Work out the finished part from the listing and answer in its coordinate system (mm). A direction names the side the tool comes from. Round coordinates to 2 decimals unless told otherwise and drop trailing zeros. Loops run counter-clockwise (first coordinate to the right, second up) from the corner with the lowest first, then second, coordinate; pieces in that order, holes last. Notation, with made-up numbers: (-10.75, 74) - (11.25, 74) arc R30 ccw to (11.25, 105) - close; hole circle Ø3 at (54.25, 85). An arc over 180 degrees is marked (long way). Return JSON: item names as keys, results as strings.
from build123d import *

# Parameters (mm, degrees)
SKETCH_1_W          = 100
SKETCH_1_H          = 11.5
EXTRUDE_1_DEPTH     = 3
SKETCH_2_W          = 2.5
SKETCH_2_H          = 11.5
EXTRUDE_2_DEPTH     = 26
SKETCH_3_W          = 2.5
SKETCH_3_H          = 11.5
EXTRUDE_3_DEPTH     = 20
SKETCH_6_W          = 2.5
SKETCH_6_H          = 16.5
EXTRUDE_4_DEPTH     = 8
CUT_EXTRUDE_1_DEPTH = 101


with BuildPart() as part:
    # 草图1 → 凸台-拉伸1 (new body)
    with BuildSketch(Plane(origin=(0, 0, 0), x_dir=(1, 0, 0), z_dir=(0, 1, 0))):
        with Locations((50, 5.75)):
            Rectangle(SKETCH_1_W, SKETCH_1_H)
    extrude(amount=EXTRUDE_1_DEPTH)

    # 草图2 → 凸台-拉伸2 (add)
    with BuildSketch(Plane(origin=(0, 3, 0), x_dir=(1, 0, 0), z_dir=(0, 1, 0))):
        with Locations((1.25, 5.75)):
            Rectangle(SKETCH_2_W, SKETCH_2_H)
        with Locations((98.75, 5.75)):
            Rectangle(SKETCH_2_W, SKETCH_2_H)
    extrude(amount=EXTRUDE_2_DEPTH)

    # 草图3 → 凸台-拉伸3 (add)
    with BuildSketch(Plane(origin=(0, 3, 0), x_dir=(1, 0, 0), z_dir=(0, 1, 0))):
        with Locations((22.25, 5.75)):
            Rectangle(SKETCH_3_W, SKETCH_3_H)
        with Locations((77.75, 5.75)):
            Rectangle(SKETCH_3_W, SKETCH_3_H)
    extrude(amount=EXTRUDE_3_DEPTH)

    # 草图6 → 凸台-拉伸4 (add)
    with BuildSketch(Plane(origin=(0, 29, 0), x_dir=(1, 0, 0), z_dir=(0, 1, 0))):
        with Locations((1.25, 5.75)):
            Rectangle(SKETCH_6_W, SKETCH_6_H)
        with Locations((98.75, 5.75)):
            Rectangle(SKETCH_6_W, SKETCH_6_H)
    extrude(amount=EXTRUDE_4_DEPTH)

    # 草图5 → 切除-拉伸1 (cut, through all)
    with BuildSketch(Plane(origin=(100, 0, 0), x_dir=(0, 0, -1), z_dir=(1, 0, 0))):
        Polygon((8.25, 31.165063509), (7, 33.330127019), (4.5, 33.330127019), (3.25, 31.165063509), (4.5, 29), (7, 29), align=None)
    extrude(amount=-CUT_EXTRUDE_1_DEPTH, mode=Mode.SUBTRACT)


solid = part.part
1) Section B-B (z = -9.5) is taken. Give the vertices of the cut face in (x, y), and give its area (3 significant figures).
Verdict:
{"outline": "(0, 0) - (100, 0) - (100, 37) - (97.5, 37) - (97.5, 3) - (79, 3) - (79, 23) - (76.5, 23) - (76.5, 3) - (23.5, 3) - (23.5, 23) - (21, 23) - (21, 3) - (2.5, 3) - (2.5, 37) - (0, 37) - close", "area": "570 mm2"}
2) Section A-A (y = 34.5) is taken. Give the vertices of the cut face in (x, z).
Verdict:
{"outline": "(0, -14) - (2.5, -14) - (2.5, 2.5) - (0, 2.5) - close; (97.5, -14) - (100, -14) - (100, 2.5) - (97.5, 2.5) - close"}
3) Section C-C (y = 13) is taken. Give the vertices of the cut face in (x, z).
Verdict:
{"outline": "(0, -11.5) - (2.5, -11.5) - (2.5, 0) - (0, 0) - close; (21, -11.5) - (23.5, -11.5) - (23.5, 0) - (21, 0) - close; (76.5, -11.5) - (79, -11.5) - (79, 0) - (76.5, 0) - close; (97.5, -11.5) - (100, -11.5) - (100, 0) - (97.5, 0) - close"}
4) Find the intervals of material crossed by L1, parallel to X at y = 16.5, z = -0.5; L2, parallel to X at y = 31.5, z = -9.25; L3, parallel to Y at x = 30.5, z = -7.25, in increasing order.
Verdict:
{"L1": "x = 0 to 2.5, 21 to 23.5, 76.5 to 79, 97.5 to 100", "L2": "x = 0 to 2.5, 97.5 to 100", "L3": "y = 0 to 3"}
5) A tool of negligible diameter and unlimited length cuts with its end or side. For faces 3 (the flat face through (88, 3, -6)), 4 (the flat face through (1.267, 32.232, -7.634)), 5 (the flat face through (99, 29, -13)), from which of +Z, -Z, +X, -X, +Y, -Y can it reach the whole face along a straight path? Write none if from no direction.
Verdict:
{"face 3": "+Z, -Z, +Y", "face 4": "+X, -X", "face 5": "-Z, +X, -X, -Y"}
6) Flat-ended cylindrical pins translate along their axes: pin 1 (10 mm diameter, centred on x = 30, y = 20, fed in from +Z); pin 2 (6 mm diameter, centred on x = 15.5, z = -6.5, fed in from +Y); pin 3 (0.8 mm diameter, centred on x = 22, z = -6, fed in from +Y); pin 4 (0.8 mm diameter, centred on x = 99, z = -12.5, fed in from -Y). Find the tip coordinate at first contact, or state that the pin passes through.
Verdict:
{"pin 1": "passes through", "pin 2": "stops at y = 3", "pin 3": "stops at y = 23", "pin 4": "stops at y = 29"}
7) Section D-D (x = 66.5) is taken. Give the vertices of the cut face in (y, z), and give its area (3 significant figures).
Verdict:
{"outline": "(0, -11.5) - (3, -11.5) - (3, 0) - (0, 0) - close", "area": "34.5 mm2"}
8) Determine the mould class of faces 1 (the flat face through (49.8, 2.6, 0)), 2 (the flat face through (12, 3, -6)) for opening direction X: pulls with the +X half, pulls with the -X half, needs draft (parallel to the pull), parting line crosses it, or undercut.
Verdict:
{"face 1": "needs draft", "face 2": "undercut"}
